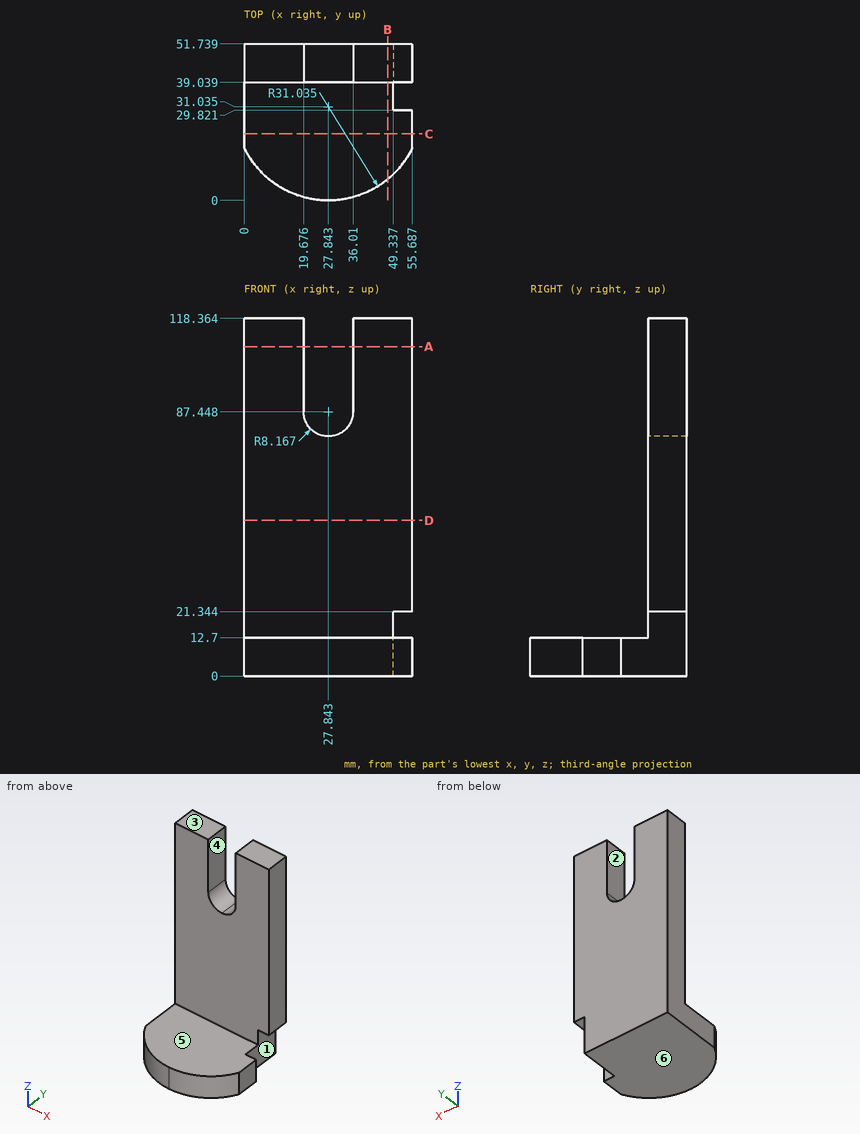
Verification items for this drawing (mm, ordinates from the low corner). A direction names the side the tool comes from. Round coordinates to 2 decimals unless told otherwise and drop trailing zeros. Order: outer loops, then holes, each group sorted by start corner. A loop starts at its lowest first (then second) coordinate and runs counter-clockwise, first axis right, second up. Notation, with made-up numbers: M -26,46 L 29,46 A35 ccw 29,82 Z; hole C 36,31 d2. An arc over 180 degrees is marked long. Answer in a Markdown table with one row per item. Add a question column.
Item 1: Material ranges on L1, parallel to Y at x = 42, z = 24; L2, parallel to Z at x = 44.5, y = 18.5; L3, parallel to X at y = 39.5, z = 87.5, recorded low to high. Write a range as [from, to].
Item 2: Draft check along X on the marked faces 1, 2 and 3. Enter one of: released by +X, released by -X, zero draft, split by the parting line, or undercut.
Item 3: Sectioned sample at A-A, the plane z = 109. Enter the section's corners in (x, y).
Item 4: Set-up check for the marked faces 4, 5 and 6: record each of +Z, -Z, +X, -X, +Y, -Y from which the full face is reachable in a straight line by a thin tool's end or side.
Item 5: Depth check by flat-ended pin: pin 1 Ø10 at (x, y) = (15, 22) entering from +Z; pin 2 Ø1.9 at (x, z) = (53.5, 9) entering from +Y; pin 3 Ø1.9 at (x, y) = (51, 47.5) entering from -Z. Enter the tip coordinate at first touch or a pass-through.
Item 6: Sectioned sample at C-C, the plane y = 22. Enter the section's corners in (x, z).
Item 7: Sectioned sample at B-B, the plane x = 47.5. Enter the section's corners in (y, z).
Item 8: Sectioned sample at D-D, the plane z = 51.5. Enter the section's corners in (x, y).
Filled in:
| question | item | result |
|---|---|---|
| 1 | L1 | y = [39.04, 51.74] |
| 1 | L2 | z = [0, 12.7] |
| 1 | L3 | x = [0, 19.68], [36.01, 55.69] |
| 2 | face 1 | released by +X |
| 2 | face 2 | undercut |
| 2 | face 3 | zero draft |
| 3 | outline | M 0,39.04 L 19.68,39.04 L 19.68,51.74 L 0,51.74 Z; M 36.01,39.04 L 55.69,39.04 L 55.69,51.74 L 36.01,51.74 Z |
| 4 | face 4 | +Z, +Y, -Y |
| 4 | face 5 | +Z, +X, -X, -Y |
| 4 | face 6 | -Z, +X, -X, +Y, -Y |
| 5 | pin 1 | stops at z = 12.7 |
| 5 | pin 2 | stops at y = 29.82 |
| 5 | pin 3 | stops at z = 21.34 |
| 6 | outline | M 0,0 L 55.69,0 L 55.69,12.7 L 0,12.7 Z |
| 7 | outline | M 7.02,0 L 51.74,0 L 51.74,118.36 L 39.04,118.36 L 39.04,12.7 L 7.02,12.7 Z |
| 8 | outline | M 0,39.04 L 55.69,39.04 L 55.69,51.74 L 0,51.74 Z |
